Verification items for the finished model (mm, model axes). Face numbers are marked on the shaded views. A direction names the side the tool comes from. Round coordinates to 2 decimals unless told otherwise and drop trailing zeros. Order: outer loops, then holes, each group sorted by start corner. A loop starts at its lowest first (then second) coordinate and runs counter-clockwise, first axis right, second up. Notation, with made-up numbers: (-18.5, -20) -> (34.5, -20) arc R11 ccw to (34.5, -7) -> close; hole circle Ø4 at (29, 59.25). An arc over 180 degrees is marked (long way). Put each result on its own line as item: value.
from build123d import *

# Parameters (mm, degrees)
BOSS_EXTRUDE2_DEPTH   = 101.6
SKETCH14_W            = 12.7
SKETCH14_H            = 13.97
BOSS_EXTRUDE3_DEPTH   = 20.32
F_6_CLEARANCE_HOLE1_D = 4.3053
SKETCH8_W             = 8.382
SKETCH8_H             = 9.144
CUT_EXTRUDE2_DEPTH    = 2.794
FILLET1_R             = 2.54


with BuildPart() as part:
    # Sketch3 → Boss-Extrude2 (new body)
    with BuildSketch(Plane(origin=(0, 0, 0), x_dir=(0, 0, -1), z_dir=(1, 0, 0))):
        with BuildLine():
            Line((40.3225, 19.05), (50.8, 19.05))
            Line((50.8, 19.05), (50.8, 0))
            Line((50.8, 0), (0, 0))
            Line((0, 0), (0, 19.05))
            Line((0, 19.05), (10.4775, 19.05))
            ThreePointArc((10.4775, 19.05), (25.4, 4.1275), (40.3225, 19.05))
        make_face()
    extrude(amount=BOSS_EXTRUDE2_DEPTH)

    # Sketch14 → Boss-Extrude3 (add)
    # profile 1 of 2: a face of its own
    with BuildSketch(Plane(origin=(0, 0, -35.56), x_dir=(-1, 0, 0), z_dir=(0, 0, -1))):
        with Locations((-69.85, -6.985)):
            Rectangle(SKETCH14_W, SKETCH14_H)
        with BuildLine():
            Line((-66.675, -5.08), (-66.675, -8.89))
            ThreePointArc((-66.675, -8.89), (-69.85, -12.065), (-73.025, -8.89))
            Line((-73.025, -8.89), (-73.025, -5.08))
            ThreePointArc((-73.025, -5.08), (-69.85, -1.905), (-66.675, -5.08))
        make_face(mode=Mode.SUBTRACT)
    # profile 2 of 2: a face of its own
    with BuildSketch(Plane(origin=(0, 0, -35.56), x_dir=(-1, 0, 0), z_dir=(0, 0, -1))):
        with Locations((-31.75, -6.985)):
            Rectangle(SKETCH14_W, SKETCH14_H)
        with BuildLine():
            Line((-28.575, -5.08), (-28.575, -8.89))
            ThreePointArc((-28.575, -8.89), (-31.75, -12.065), (-34.925, -8.89))
            Line((-34.925, -8.89), (-34.925, -5.08))
            ThreePointArc((-34.925, -5.08), (-31.75, -1.905), (-28.575, -5.08))
        make_face(mode=Mode.SUBTRACT)
    extrude(amount=-BOSS_EXTRUDE3_DEPTH)

    # #6 Clearance Hole1 (through all)
    with Locations(Plane(origin=(0, 19.05, 0), x_dir=(1, 0, 0), z_dir=(0, 1, 0))):
        with Locations((50.8, 5.08), (50.8, 45.72)):
            Hole(F_6_CLEARANCE_HOLE1_D / 2)

    # Sketch8 → Cut-Extrude2 (cut)
    with BuildSketch(Plane(origin=(0, 13.97, 0), x_dir=(1, 0, 0), z_dir=(0, 1, 0))):
        with Locations((50.8, 4.572)):
            Rectangle(SKETCH8_W, SKETCH8_H)
        with Locations((50.8, 46.228)):
            Rectangle(SKETCH8_W, SKETCH8_H)
    extrude(amount=CUT_EXTRUDE2_DEPTH, mode=Mode.SUBTRACT)

    # Fillet1
    # the kernel refuses this fillet: 2.54 mm, written as the material it adds along each edge
    with BuildSketch(Plane(origin=(63.5, 0, -35.56), x_dir=(-1, 0, 0), z_dir=(0, 0, 1)), Plane(origin=(25.4, 0, -35.56), x_dir=(-1, 0, 0), z_dir=(0, 0, 1))) as fillet1_piece_1:
        with BuildLine():
            CenterArc((FILLET1_R, FILLET1_R), FILLET1_R, 180, 90)
            Line((0, FILLET1_R), (0, 0))
            Line((0, 0), (FILLET1_R, 0))
        make_face()
    extrude(amount=20.32)
    with BuildSketch(Plane(origin=(76.2, 0, -35.56), x_dir=(1, 0, 0), z_dir=(0, 0, 1)), Plane(origin=(38.1, 0, -35.56), x_dir=(1, 0, 0), z_dir=(0, 0, 1))) as fillet1_piece_2:
        with BuildLine():
            CenterArc((FILLET1_R, -FILLET1_R), FILLET1_R, 90, 90)
            Line((0, -FILLET1_R), (0, 0))
            Line((0, 0), (FILLET1_R, 0))
        make_face()
    extrude(amount=20.32)
    # the kernel refuses this fillet: 2.54 mm, written as the material it takes off along each edge
    with BuildSketch(Plane(origin=(2.54, 2.54, -48.26), x_dir=(-1, 0, 0), z_dir=(0, 0, -1))) as fillet1_2_piece_1_section:
        Polygon((0, 0), (FILLET1_R, 0), (FILLET1_R, -FILLET1_R), (0, -FILLET1_R), align=None)
    fillet1_2_piece_1 = extrude(amount=FILLET1_R, mode=Mode.PRIVATE)
    fillet1_2_piece_1 = fillet1_2_piece_1 - Plane(origin=(2.54, 2.54, -48.26), x_dir=(0.7071067811865475, 0.7071067811865475, 0), z_dir=(0, 0, -1)) * Sphere(FILLET1_R, mode=Mode.PRIVATE)
    add(fillet1_2_piece_1, mode=Mode.SUBTRACT)
    with BuildSketch(Plane(origin=(99.06, 2.54, -48.26), x_dir=(1, 0, 0), z_dir=(0, 0, -1))) as fillet1_2_piece_2_section:
        Polygon((0, 0), (FILLET1_R, 0), (FILLET1_R, FILLET1_R), (0, FILLET1_R), align=None)
    fillet1_2_piece_2 = extrude(amount=FILLET1_R, mode=Mode.PRIVATE)
    fillet1_2_piece_2 = fillet1_2_piece_2 - Plane(origin=(99.06, 2.54, -48.26), x_dir=(-0.7071067811865475, 0.7071067811865475, 0), z_dir=(0, 0, -1)) * Sphere(FILLET1_R, mode=Mode.PRIVATE)
    add(fillet1_2_piece_2, mode=Mode.SUBTRACT)
    with BuildSketch(Plane(origin=(2.54, 2.54, -2.54), x_dir=(0, 0, 1), z_dir=(-1, 0, 0))) as fillet1_2_piece_3_section:
        Polygon((0, 0), (FILLET1_R, 0), (FILLET1_R, -FILLET1_R), (0, -FILLET1_R), align=None)
    fillet1_2_piece_3 = extrude(amount=FILLET1_R, mode=Mode.PRIVATE)
    fillet1_2_piece_3 = fillet1_2_piece_3 - Plane(origin=(2.54, 2.54, -2.54), x_dir=(0, 0.7071067811865475, -0.7071067811865475), z_dir=(-1, 0, 0)) * Sphere(FILLET1_R, mode=Mode.PRIVATE)
    add(fillet1_2_piece_3, mode=Mode.SUBTRACT)
    with BuildSketch(Plane(origin=(99.06, 2.54, -2.54), x_dir=(0, 0, 1), z_dir=(1, 0, 0))) as fillet1_2_piece_4_section:
        Polygon((0, 0), (FILLET1_R, 0), (FILLET1_R, FILLET1_R), (0, FILLET1_R), align=None)
    fillet1_2_piece_4 = extrude(amount=FILLET1_R, mode=Mode.PRIVATE)
    fillet1_2_piece_4 = fillet1_2_piece_4 - Plane(origin=(99.06, 2.54, -2.54), x_dir=(0, 0.7071067811865475, -0.7071067811865475), z_dir=(1, 0, 0)) * Sphere(FILLET1_R, mode=Mode.PRIVATE)
    add(fillet1_2_piece_4, mode=Mode.SUBTRACT)
    with BuildSketch(Plane(origin=(2.54, 0, -50.8), x_dir=(0, 0, 1), z_dir=(1, 0, 0))) as fillet1_2_piece_5:
        with BuildLine():
            CenterArc((FILLET1_R, -FILLET1_R), FILLET1_R, 90, 90)
            Line((0, -FILLET1_R), (0, 0))
            Line((0, 0), (FILLET1_R, 0))
        make_face()
    extrude(amount=96.52, mode=Mode.SUBTRACT)
    with BuildSketch(Plane(origin=(2.54, 0, 0), x_dir=(0, 0, -1), z_dir=(1, 0, 0))) as fillet1_2_piece_6:
        with BuildLine():
            CenterArc((FILLET1_R, FILLET1_R), FILLET1_R, 180, 90)
            Line((0, FILLET1_R), (0, 0))
            Line((0, 0), (FILLET1_R, 0))
        make_face()
    extrude(amount=96.52, mode=Mode.SUBTRACT)
    with BuildSketch(Plane(origin=(101.6, 25.4, -50.8), x_dir=(-1, 0, 0), z_dir=(0, -1, 0)), Plane(origin=(101.6, 2.54, 0), x_dir=(-1, 0, 0), z_dir=(0, 1, 0))) as fillet1_2_piece_7:
        with BuildLine():
            CenterArc((FILLET1_R, -FILLET1_R), FILLET1_R, 90, 90)
            Line((0, -FILLET1_R), (0, 0))
            Line((0, 0), (FILLET1_R, 0))
        make_face()
    extrude(amount=22.86, mode=Mode.SUBTRACT)
    with BuildSketch(Plane(origin=(101.6, 19.05, -33.9725), x_dir=(-1, 0, 0), z_dir=(0, 0, -1)), Plane(origin=(101.6, 19.05, 6.35), x_dir=(-1, 0, 0), z_dir=(0, 0, -1))) as fillet1_2_piece_8:
        with BuildLine():
            CenterArc((FILLET1_R, -FILLET1_R), FILLET1_R, 90, 90)
            Line((0, -FILLET1_R), (0, 0))
            Line((0, 0), (FILLET1_R, 0))
        make_face()
    extrude(amount=23.1775, mode=Mode.SUBTRACT)
    with BuildSketch(Plane(origin=(101.6, 19.05, -25.4), x_dir=(0, 0.4134285279773088, 0.9105365738148663), z_dir=(0, 0.9105365738148663, -0.4134285279773088))) as fillet1_2_piece_9:
        with BuildLine():
            CenterArc((14.9225 + FILLET1_R, -FILLET1_R), FILLET1_R, 90, 90)
            Line((14.9225, -FILLET1_R), (14.9225, 0))
            Line((14.9225, 0), (14.9225 + FILLET1_R, 0))
        make_face()
    revolve(axis=Axis((101.6, 19.05, -25.4), (1, 0, 0)), revolution_arc=228.840784647, mode=Mode.SUBTRACT)
    with BuildSketch(Plane(origin=(63.5, -13.97, -41.91), x_dir=(1, 0, 0), z_dir=(0, 0, 1)), Plane(origin=(76.2, -13.97, -41.91), x_dir=(0, 1, 0), z_dir=(0, 0, 1)), Plane(origin=(25.4, -13.97, -41.91), x_dir=(1, 0, 0), z_dir=(0, 0, 1)), Plane(origin=(38.1, -13.97, -41.91), x_dir=(0, 1, 0), z_dir=(0, 0, 1))) as fillet1_2_piece_10:
        with BuildLine():
            CenterArc((FILLET1_R, FILLET1_R), FILLET1_R, 180, 90)
            Line((0, FILLET1_R), (0, 0))
            Line((0, 0), (FILLET1_R, 0))
        make_face()
    extrude(amount=33.02, mode=Mode.SUBTRACT)
    with BuildSketch(Plane(origin=(0, 19.05, 6.35), x_dir=(1, 0, 0), z_dir=(0, 0, -1)), Plane(origin=(0, 19.05, -33.9725), x_dir=(1, 0, 0), z_dir=(0, 0, -1))) as fillet1_2_piece_11:
        with BuildLine():
            CenterArc((FILLET1_R, FILLET1_R), FILLET1_R, 180, 90)
            Line((0, FILLET1_R), (0, 0))
            Line((0, 0), (FILLET1_R, 0))
        make_face()
    extrude(amount=23.1775, mode=Mode.SUBTRACT)
    with BuildSketch(Plane(origin=(0, 19.05, -25.4), x_dir=(0, 0.4134285279773076, 0.9105365738148669), z_dir=(0, 0.9105365738148669, -0.4134285279773076))) as fillet1_2_piece_12:
        with BuildLine():
            CenterArc((14.9225 + FILLET1_R, FILLET1_R), FILLET1_R, 180, 90)
            Line((14.9225, FILLET1_R), (14.9225, 0))
            Line((14.9225, 0), (14.9225 + FILLET1_R, 0))
        make_face()
    revolve(axis=Axis((0, 19.05, -25.4), (1, 0, 0)), revolution_arc=228.840784647, mode=Mode.SUBTRACT)
    with BuildSketch(Plane(origin=(0, 25.4, -50.8), x_dir=(1, 0, 0), z_dir=(0, -1, 0)), Plane(origin=(0, 2.54, 0), x_dir=(1, 0, 0), z_dir=(0, 1, 0))) as fillet1_2_piece_13:
        with BuildLine():
            CenterArc((FILLET1_R, FILLET1_R), FILLET1_R, 180, 90)
            Line((0, FILLET1_R), (0, 0))
            Line((0, 0), (FILLET1_R, 0))
        make_face()
    extrude(amount=22.86, mode=Mode.SUBTRACT)
    with BuildSketch(Plane(origin=(0, 0, -48.26), x_dir=(1, 0, 0), z_dir=(0, 0, 1))) as fillet1_2_piece_14:
        with BuildLine():
            CenterArc((FILLET1_R, FILLET1_R), FILLET1_R, 180, 90)
            Line((0, FILLET1_R), (0, 0))
            Line((0, 0), (FILLET1_R, 0))
        make_face()
    extrude(amount=45.72, mode=Mode.SUBTRACT)
    with BuildSketch(Plane(origin=(101.6, 0, -48.26), x_dir=(-1, 0, 0), z_dir=(0, 0, 1))) as fillet1_2_piece_15:
        with BuildLine():
            CenterArc((FILLET1_R, -FILLET1_R), FILLET1_R, 90, 90)
            Line((0, -FILLET1_R), (0, 0))
            Line((0, 0), (FILLET1_R, 0))
        make_face()
    extrude(amount=45.72, mode=Mode.SUBTRACT)


solid = part.part
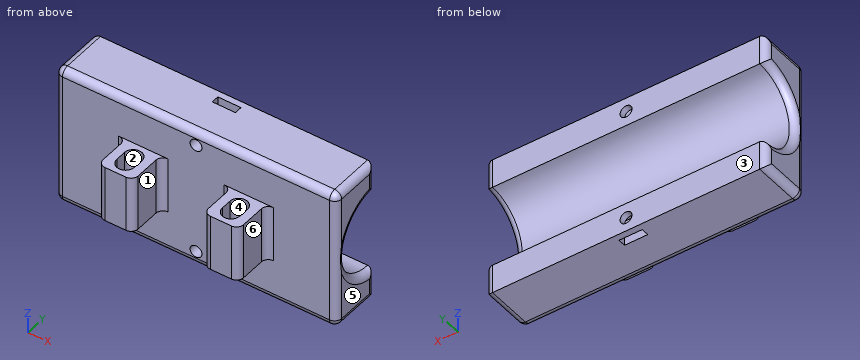
Item 1: Section check B-B on z = -45.72. Record the boundary of the cut face in (x, y), then the cut area to 3 significant figures.
Check sheet entries:
outline: (0, 2.54) arc R2.54 ccw to (2.54, 0) -> (48.65, 0) -> (48.65, 13.97) -> (46.61, 13.97) -> (46.61, 16.76) -> (48.65, 16.76) -> (48.65, 19.05) -> (2.54, 19.05) arc R2.54 ccw to (0, 16.51) -> close; (52.95, 0) -> (99.06, 0) arc R2.54 ccw to (101.6, 2.54) -> (101.6, 16.51) arc R2.54 ccw to (99.06, 19.05) -> (52.95, 19.05) -> (52.95, 16.76) -> (54.99, 16.76) -> (54.99, 13.97) -> (52.95, 13.97) -> close
area: 1,840 mm^2
Item 2: Gauge pin test, flat ends, axial feed: pin 1 Ø5 at (x, z) = (37.5, -24) entering from -Y; pin 2 Ø10 at (y, z) = (-5.5, -27.5) entering from +X; pin 3 Ø6.5 at (x, z) = (49, -46.5) entering from -Y; pin 4 Ø10 at (y, z) = (-3.5, -9) entering from -X. Record the tip position at first contact, or that the pin passes through.
Check sheet entries:
pin 1: stops at y = -13.97
pin 2: stops at x = 77.23
pin 3: stops at y = 0
pin 4: stops at x = 0.22
Item 3: Section check C-C on x = 50.8. State how many separate pieces and enclosed holes the cut face has, then the cut area to 3 significant figures.
Check sheet entries:
separate pieces: 5
enclosed holes: 0
area: 424 mm^2
Item 4: Tool access check on the marked faces 4, 5 and 6. Record the directions out of +Z, -Z, +X, -X, +Y, -Y that give a thin tool (end or side, any length) a straight path to the whole face; none if there is none.
Check sheet entries:
face 4: +Z, -Z
face 5: +Z, -Z, +X, +Y, -Y
face 6: +Z, -Z, +X, -Y
Item 5: Release check for a two-part mould opening along Y. For the marked faces 1, 2 and 3 record: +Y half, -Y half, draft (parallel to the pull), parting line (faces both ways), or undercut.
Check sheet entries:
face 1: draft
face 2: undercut
face 3: +Y half
Item 6: Material ranges on L1, parallel to X at y = -6.5, z = -16 (3 decimals); L2, parallel to Z at x = 50.8, y = 6.5; L3, parallel to Z at x = 50.8, y = 18.05, recorded low to high. Write a range as [from, to].
Check sheet entries:
L1: x = [25.4, 28.575], [34.925, 38.1], [63.5, 66.675], [73.025, 76.2]
L2: z = [-50.8, -47.87], [-43.57, -33.47], [-17.33, -7.23], [-2.93, 0]
L3: z = [-50.8, -47.87], [-43.57, -40.29], [-10.51, -7.23], [-2.93, 0]
